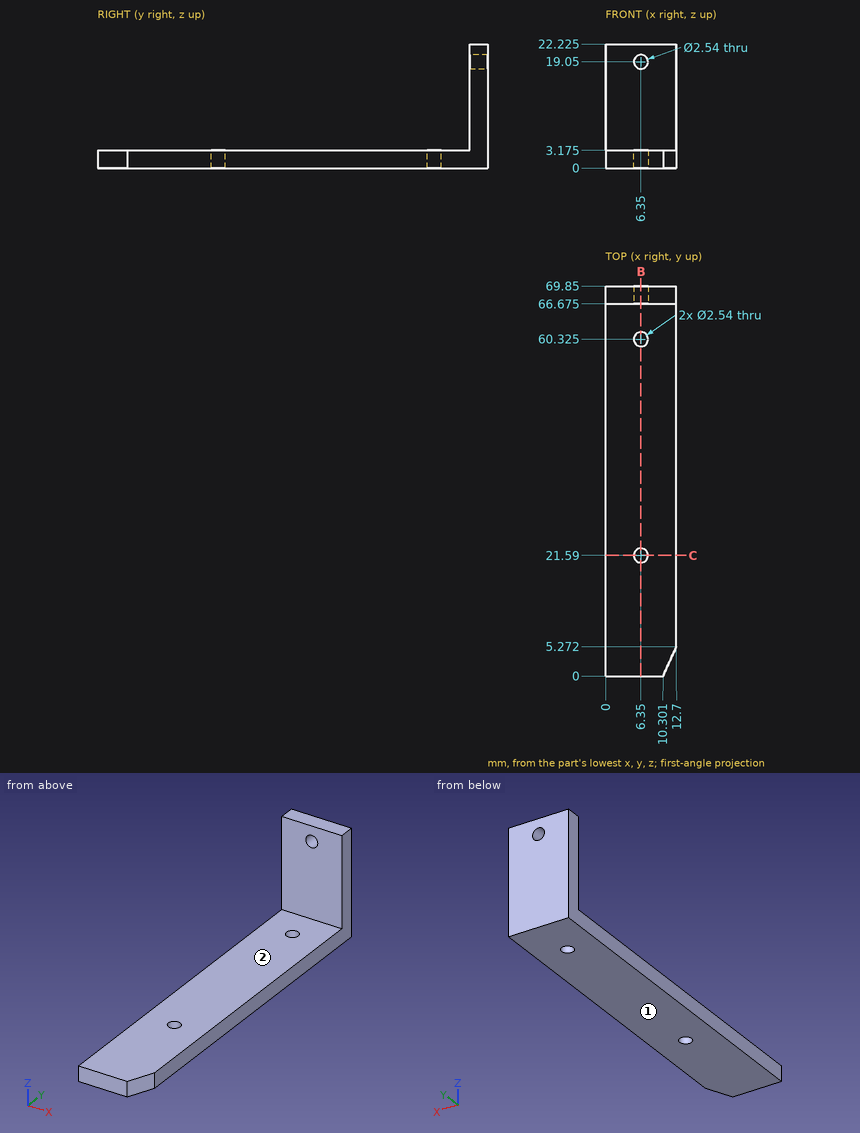
Design review of the part shown in the three views and the two pictorial views. Dimensions are in mm from the part's minimum x, y and z. A direction names the side the tool comes from. Give positions to 0.01 mm unless a question says otherwise; leave off trailing zeros. Loops run counter-clockwise (first coordinate to the right, second up) from the corner with the lowest first, then second, coordinate; pieces in that order, holes last. Notation, with made-up numbers: (-18.5, 66.5) - (31.5, 66.5) arc R31 cw to (31.5, 100.5) - close; hole circle Ø7 at (77.25, 61.25). An arc over 180 degrees is marked (long way). Write item = value, one per line.
1) To check wall thickness, follow line 1 (X direction, y = 68.55, z = 19.05); line 2 (Z direction, x = 5.5, y = 50) (1 decimal). State the ranges of each line that lie inside material, in increasing order.
Result sheet:
line_1 = 0 to 5.08, 7.62 to 12.7
line_2 = 0 to 3.2
2) Take a section at B-B on x = 6.35. Count the separate pieces of the cut face and the enclosed holes in it, and give its area (3 significant figures).
Result sheet:
separate_pieces = 4
enclosed_holes = 0
area = 258 mm2
3) Tool access review of the marked faces 1 and 2: name each direction out of +Z, -Z, +X, -X, +Y, -Y from which nothing blocks a thin tool from reaching the whole face with its end or side.
Result sheet:
face_1 = -Z, +X, -X, +Y, -Y
face_2 = +Z, +X, -X, -Y
4) Clearance check with flat-ended pins moving along their axes: pin 1 Ø4 at (x, z) = (11, 13) entering from -Y (1 decimal); pin 2 Ø5 at (y, z) = (35, 7.5) entering from +X; pin 3 Ø3 at (x, y) = (6.35, 21.59) entering from -Z. State where each tip first meets the part, or that it passes through.
Result sheet:
pin_1 = 66.7
pin_2 = through
pin_3 = 0
5) Take a section at C-C on y = 21.59. State the section outline as (x, z) points (1 decimal).
Result sheet:
outline = (0, 0) - (5.1, 0) - (5.1, 3.2) - (0, 3.2) - close; (7.6, 0) - (12.7, 0) - (12.7, 3.2) - (7.6, 3.2) - close
